Could you check a few things on this model? Use its own coordinates, in mm. A direction names the side the tool comes from. Coordinates: 2 decimals unless noted, no trailing zeros. Loops run counter-clockwise (first coordinate to the right, second up) from the corner with the lowest first, then second, coordinate; pieces in that order, holes last. Notation, with made-up numbers: (38.25, -7.75) - (47.25, -7.75) arc R24 ccw to (47.25, 21.25) - close; hole circle Ø7 at (-20.75, -34). An arc over 180 degrees is marked (long way). One line per question, with ' | ' between items. Start each with the question number.
1. I'm going to push flat-ended pins straight in: P1, Ø6, axis at x = -182.63, z = -37.83, coming from the +Y side; P2, Ø2.5, axis at y = 2, z = 49.5, coming from the +X side; P3, Ø2.5, axis at y = 3, z = -25.5, coming from the +X side; P4, Ø3.5, axis at x = -141.45, z = 26.33, coming from the +Y side. Where does each tip first touch, or does it pass through?
2. I want a section at D-D, the plane y = 4.05. Count the separate pieces of the cut face and the enclosed holes in it, then the cut area to 3 significant figures.
3. I want a section at C-C, the plane z = 95.5. Write out the boundary of the cut face in (x, y) (3 decimals), then the cut area to 3 significant figures.
4. Please list where these lines run through material, in increasing order: L1, parallel to Z at x = -172.5, y = 2.9; L2, parallel to X at y = 3.7, z = 83 (3 decimals); L3, parallel to Z at x = -156, y = 1.6. Write a range as [from, to].
5. Which directions (+Z, -Z, +X, -X, +Y, -Y) give clear straight access to the entire face, cutting with the end or side of a thin tool? Please do faces 4 (the flat face through (-201.613, 3, -17)), 5 (the flat face through (-215.9, 3, 86)), 6 (the flat face through (-172, 3, -50.8)), 7 (the flat face through (-141.288, 3, -18)), 8 (the flat face through (-193.675, 3, 68)).
6. I want a section at A-A, the plane x = -176. Write out the boundary of the cut face in (y, z), then the cut area to 3 significant figures.
7. We'd pull the mould along Z, two halves only. Please class faces 1 (the cylindrical face through (-199.76, 2.5, 27.4)), 2 (the flat face through (-171, 3, 110.889)), 3 (the flat face through (-127, 3, 85)): pulls with the +Z half, pulls with the -Z half, needs draft (parallel to the pull), parting line crosses it, or undercut.
8. I want a section at B-B, the plane z = -12. Write out the boundary of the cut face in (x, y) (1 decimal).
from build123d import *

# Parameters (mm, degrees)
SKETCH1_R           = 2.000308567
SKETCH1_R_2         = 2.000222439
SKETCH1_R_3         = 1.777841526
SKETCH1_R_4         = 1.904793294
SKETCH1_R_5         = 1.777669271
SKETCH1_R_6         = 1.777927653
SKETCH1_R_7         = 1.904965549
SKETCH1_R_8         = 1.77801378
SKETCH1_W           = 44.45
SKETCH1_H           = 27.635522461
BOSS_EXTRUDE2_DEPTH = 5.08


with BuildPart() as part:
    # Sketch1 → Boss-Extrude2 (new body)
    with BuildSketch(Plane(origin=(0, 0, 0), x_dir=(1, 0, 0), z_dir=(0, 1, 0))):
        with BuildLine():
            Line((-201.612672255, -11.699372016), (-201.612672255, 47.168869358))
            add(Edge.make_bspline(
                [(-201.612672255, 47.168869358), (-201.612672255, 49.174431695), (-199.986931695, 50.8), (-197.981369358, 50.8)],
                knots=[1, 1, 1, 1, 2, 2, 2, 2], degree=3))
            Line((-197.981369358, 50.8), (-144.918975152, 50.8))
            add(Edge.make_bspline(
                [(-144.918975152, 50.8), (-142.913585069, 50.8), (-141.2875, 49.174431695), (-141.2875, 47.168869358)],
                knots=[3, 3, 3, 3, 4, 4, 4, 4], degree=3))
            Line((-141.2875, 47.168869358), (-141.2875, -11.699372016))
            add(Edge.make_bspline(
                [(-141.2875, -11.699372016), (-141.2875, -20.416152615), (-127, -44.166985406), (-127, -64.33991428)],
                knots=[5, 5, 5, 5, 6, 6, 6, 6], degree=3))
            Line((-127, -64.33991428), (-127, -106.638107639))
            add(Edge.make_bspline(
                [(-127, -106.638107639), (-127, -108.986284722), (-128.800062391, -110.889355469), (-131.020426432, -110.889355469)],
                knots=[7, 7, 7, 7, 8, 8, 8, 8], degree=3))
            Line((-131.020426432, -110.889355469), (-211.879229058, -110.889355469))
            add(Edge.make_bspline(
                [(-211.879229058, -110.889355469), (-214.099765354, -110.889355469), (-215.9, -108.986284722), (-215.9, -106.638107639)],
                knots=[9, 9, 9, 9, 10, 10, 10, 10], degree=3))
            Line((-215.9, -106.638107639), (-215.9, -64.33991428))
            add(Edge.make_bspline(
                [(-215.9, -64.33991428), (-215.9, -44.166985406), (-201.612672255, -20.416152615), (-201.612672255, -11.699372016)],
                knots=[11, 11, 11, 11, 12, 12, 12, 12], degree=3))
        make_face()
        with Locations(Location((-201.447479926, -44.309353977, 0), (0, 0, 270))):
            Circle(SKETCH1_R, mode=Mode.SUBTRACT)
        with Locations(Location((-141.452864583, -44.309353977, 0), (0, 0, 270))):
            Circle(SKETCH1_R, mode=Mode.SUBTRACT)
        with Locations(Location((-141.452864583, -26.325869412, 0), (0, 0, 270))):
            Circle(SKETCH1_R_2, mode=Mode.SUBTRACT)
        with Locations(Location((-193.675, -8.524372016, 0), (0, 0, 270))):
            Circle(SKETCH1_R_3, mode=Mode.SUBTRACT)
        with Locations(Location((-160.274110243, -14.239440918, 0), (0, 0, 270))):
            Circle(SKETCH1_R_4, mode=Mode.SUBTRACT)
        with Locations(Location((-149.225, -8.524372016, 0), (0, 0, 270))):
            Circle(SKETCH1_R_5, mode=Mode.SUBTRACT)
        with Locations(Location((-193.674913873, 32.115696886, 0), (0, 0, 270))):
            Circle(SKETCH1_R_6, mode=Mode.SUBTRACT)
        with Locations(Location((-182.626062012, 37.830765788, 0), (0, 0, 270))):
            Circle(SKETCH1_R_7, mode=Mode.SUBTRACT)
        with Locations(Location((-160.273937988, 37.830765788, 0), (0, 0, 270))):
            Circle(SKETCH1_R_7, mode=Mode.SUBTRACT)
        with Locations(Location((-149.225, 32.115696886, 0), (0, 0, 270))):
            Circle(SKETCH1_R_5, mode=Mode.SUBTRACT)
        with Locations(Location((-182.626062012, -14.239440918, 0), (0, 0, 270))):
            Circle(SKETCH1_R_7, mode=Mode.SUBTRACT)
        with Locations(Location((-201.447479926, -26.325869412, 0), (0, 0, 270))):
            Circle(SKETCH1_R_2, mode=Mode.SUBTRACT)
        with Locations(Location((-211.1375, -68.026510959, 0), (0, 0, 270))):
            Circle(SKETCH1_R_8, mode=Mode.SUBTRACT)
        with Locations(Location((-131.7625, -102.951510959, 0), (0, 0, 270))):
            Circle(SKETCH1_R_8, mode=Mode.SUBTRACT)
        with Locations(Location((-211.1375, -102.951510959, 0), (0, 0, 270))):
            Circle(SKETCH1_R_8, mode=Mode.SUBTRACT)
        with Locations(Location((-131.7625, -68.026510959, 0), (0, 0, 270))):
            Circle(SKETCH1_R_8, mode=Mode.SUBTRACT)
        Polygon((-193.675, -102.951855469), (-193.675, -31.789790853), (-185.880299208, -21.022144911), (-157.698901367, -21.022144911), (-149.225, -31.789790853), (-149.225, -102.951855469), align=None, mode=Mode.SUBTRACT)
        with Locations((-171.45, 8.542458768)):
            Rectangle(SKETCH1_W, SKETCH1_H, mode=Mode.SUBTRACT)
    extrude(amount=BOSS_EXTRUDE2_DEPTH)


solid = part.part
Results are:
1) P1: stops at y = 5.08 | P2: stops at x = -128.76 | P3: stops at x = -141.29 | P4: passes through
2) separate pieces: 1 | enclosed holes: 18 | area: 6,960 mm2
3) outline: (-215.9, 0) - (-193.675, 0) - (-193.675, 5.08) - (-215.9, 5.08) - close; (-149.225, 0) - (-127, 0) - (-127, 5.08) - (-149.225, 5.08) - close | area: 226 mm2
4) L1: z = [-50.8, -22.36], [5.28, 21.02], [102.95, 110.89] | L2: x = [-215.9, -193.675], [-149.225, -127] | L3: z = [-50.8, -22.36], [5.28, 23.18], [102.95, 110.89]
5) face 4: -Z, -X, +Y, -Y | face 5: +Z, -Z, -X, +Y, -Y | face 6: -Z, +X, -X, +Y, -Y | face 7: -Z, +X, +Y, -Y | face 8: +Y, -Y
6) outline: (0, -50.8) - (5.08, -50.8) - (5.08, -22.36) - (0, -22.36) - close; (0, 5.28) - (5.08, 5.28) - (5.08, 21.02) - (0, 21.02) - close; (0, 102.95) - (5.08, 102.95) - (5.08, 110.89) - (0, 110.89) - close | area: 265 mm2
7) face 1: undercut | face 2: pulls with the +Z half | face 3: needs draft
8) outline: (-201.6, 0) - (-193.7, 0) - (-193.7, 5.1) - (-201.6, 5.1) - close; (-149.2, 0) - (-141.3, 0) - (-141.3, 5.1) - (-149.2, 5.1) - close
